Read the model definition and answer for the solid it produces. Units are mm, in the model's axes. A direction names the side the tool comes from. Round coordinates to 2 decimals unless told otherwise and drop trailing zeros. Order: outer loops, then holes, each group sorted by start corner. A loop starts at its lowest first (then second) coordinate and runs counter-clockwise, first axis right, second up.
from build123d import *

# Parameters (mm, degrees)
F0_R     = 1.5875
F0_R_2   = 3.175
F1_DEPTH = 3.048


with BuildPart() as f1:
    # F0 (on Front) → F1 (new body)
    with BuildSketch(Plane.XZ):
        with BuildLine():
            ThreePointArc((9.516015, 51.213634), (9.522753, 51.006866), (9.525, 50.8))
            ThreePointArc((9.525, 50.8), (0.006912, 41.275003), (-9.52499, 50.786176))
            Line((-9.52499, 50.786176), (-15.747385, 2.008853))
            ThreePointArc((-15.747385, 2.008853), (0.007231, 15.874998), (15.749209, 1.994506))
            Line((15.749209, 1.994506), (9.516015, 51.213634))
        make_face()
        with Locations((-4.806304, 35.006166)):
            Circle(F0_R, mode=Mode.SUBTRACT)
        with BuildLine():
            ThreePointArc((-9.52499, 50.786176), (0.006912, 41.275003), (9.525, 50.8))
            ThreePointArc((9.525, 50.8), (9.522753, 51.006866), (9.516015, 51.213634))
            ThreePointArc((9.516015, 51.213634), (-0.213776, 60.322601), (-9.52499, 50.786176))
        make_face()
        with Locations((0, 50.8)):
            Circle(F0_R_2, mode=Mode.SUBTRACT)
        with BuildLine():
            ThreePointArc((15.875, 0), (15.843521, 0.999235), (15.749209, 1.994506))
            ThreePointArc((15.749209, 1.994506), (0.007231, 15.874998), (-15.747385, 2.008853))
            ThreePointArc((-15.747385, 2.008853), (-1.006451, -15.843064), (15.875, 0))
        make_face()
        Circle(F0_R, mode=Mode.SUBTRACT)
        with BuildLine():
            Line((16.001796, 0), (15.749209, 1.994506))
            ThreePointArc((15.749209, 1.994506), (15.843521, 0.999235), (15.875, 0))
            ThreePointArc((15.875, 0), (-1.006451, -15.843064), (-15.747385, 2.008853))
            Line((-15.747385, 2.008853), (-16.003649, 0))
            Line((-16.003649, 0), (-9.461613, -62.40296))
            ThreePointArc((-9.461613, -62.40296), (0.549435, -53.99086), (9.525, -63.5))
            ThreePointArc((9.525, -63.5), (6.970557, -69.991299), (0.677344, -73.000886))
            Line((0.677344, -73.000886), (44.732405, -71.432475))
            ThreePointArc((44.732405, -71.432475), (36.5125, -63.5), (44.732405, -55.567525))
            Line((44.732405, -55.567525), (18.981753, -54.650772))
            ThreePointArc((18.981753, -54.650772), (13.27275, -51.930861), (11.354835, -45.904898))
            Line((11.354835, -45.904898), (16.001796, 0))
        make_face()
        with BuildLine():
            ThreePointArc((9.525, -63.5), (0.549435, -53.99086), (-9.461613, -62.40296))
            ThreePointArc((-9.461613, -62.40296), (-7.112487, -69.835468), (0, -73.025))
            Line((0, -73.025), (0.677344, -73.000886))
            ThreePointArc((0.677344, -73.000886), (6.970557, -69.991299), (9.525, -63.5))
        make_face()
        with Locations((0, -63.5)):
            Circle(F0_R, mode=Mode.SUBTRACT)
        with BuildLine():
            ThreePointArc((52.3875, -63.5), (50.161633, -57.98809), (44.732405, -55.567525))
            ThreePointArc((44.732405, -55.567525), (36.5125, -63.5), (44.732405, -71.432475))
            ThreePointArc((44.732405, -71.432475), (50.161633, -69.01191), (52.3875, -63.5))
        make_face()
        with Locations((44.45, -63.5)):
            Circle(F0_R, mode=Mode.SUBTRACT)
    extrude(amount=F1_DEPTH)


solid = f1.part
Q1. A cutting plane is placed at C-C, the plane z = -48.5. Give the vertices of the cut face in (x, y).
Outcome:
outline: (-10.92, -3.05) - (11.52, -3.05) - (11.52, 0) - (-10.92, 0) - close
Q2. A cutting plane is placed at B-B, the plane y = -0.55. Give the number of separate pieces and of enclosed holes in the cut face, plus the area to 3 significant figures.
Outcome:
separate pieces: 1
enclosed holes: 5
area: 3,860 mm2
Q3. A cutting plane is placed at A-A, the plane x = -4.5. Give the vertices of the cut face in (y, z), plus the area to 3 significant figures.
Outcome:
outline: (-3.05, -71.89) - (0, -71.89) - (0, 33.45) - (-3.05, 33.45) - close; (-3.05, 36.56) - (0, 36.56) - (0, 59.19) - (-3.05, 59.19) - close
area: 390 mm2
Q4. For faces 1 (the face through (-3.34, -1.5, 34.4)), 2 (the face through (13.646, -1.503, -23.274)), determine the directions among +Z, -Z, +X, -X, +Y, -Y from which every point of the face is accessible in a straight line to the end or side of a thin tool.
Outcome:
face 1: +Y, -Y
face 2: +X, +Y, -Y
Q5. Flat-ended cylindrical pins translate along their axes: pin 1 (1.5 mm diameter, centred on x = 33, y = -1.5, fed in from -Z); pin 2 (10 mm diameter, centred on x = 24.5, z = 5, fed in from +Y); pin 3 (1 mm diameter, centred on x = 21, y = -2.5, fed in from -Z); pin 4 (1.5 mm diameter, centred on x = -8.5, y = -2.5, fed in from -Z). Find the tip coordinate at first contact, or state that the pin passes through.
Outcome:
pin 1: stops at z = -71.88
pin 2: passes through
pin 3: stops at z = -72.3
pin 4: stops at z = -69.04
Q6. A cutting plane is placed at D-D, the plane z = 45. Give the vertices of the cut face in (x, y), plus the area to 3 significant figures.
Outcome:
outline: (-10.26, -3.05) - (10.3, -3.05) - (10.3, 0) - (-10.26, 0) - close
area: 62.7 mm2
Q7. Straight lines are drawn through the part: probe 1 along Z at (x, y) = (0, -1.5) (1 decimal); probe 2 along X at (y, z) = (-1.3, 34); probe 3 along X at (y, z) = (-0.2, 28). For each, find the intervals that lie inside material, in ascending order.
Outcome:
probe 1: z = -73 to -65.1, -61.9 to -1.6, 1.6 to 47.6, 54 to 60.3
probe 2: x = -11.67 to -6.03, -3.58 to 11.7
probe 3: x = -12.43 to 12.46
